```python
from build123d import *

# Parameters (mm, degrees)
SM_BASE_FLANGE_1_DEPTH = 910
SKETCH_6_W             = 17
SKETCH_6_H             = 97
CUT_EXTRUDE_1_DEPTH    = 24
SKETCH_7_W             = 101
SKETCH_7_H             = 35
CUT_EXTRUDE_2_DEPTH    = 59
CUT_EXTRUDE_3_DEPTH    = 10
SKETCH_9_R             = 3.5
SKETCH_9_R_2           = 6
CUT_EXTRUDE_3433_DEPTH = 10
SKETCH_10_R            = 3.25
SKETCH_10_R_2          = 6.5
CUT_EXTRUDE_5_DEPTH    = 10
SKETCH_11_R            = 2.5
CUT_EXTRUDE_6_DEPTH    = 10
SKETCH_12_R            = 3.25
CUT_EXTRUDE_7_DEPTH    = 10
SKETCH_13_R            = 2.5
CUT_EXTRUDE_8_DEPTH    = 10
SKETCH_16_R            = 2.5
CUT_EXTRUDE_11_DEPTH   = 10


# Sheet-metal steps are written as plain solids
with BuildPart() as part:
    # Sketch 1 → Базовая кромка1 (new, symmetric)
    with BuildSketch(Plane.XY):
        with BuildLine():
            Line((0, 0), (0, 18))
            ThreePointArc((0, 18), (-0.585786438, 19.414213562), (-2, 20))
            Line((-2, 20), (-11, 20))
            ThreePointArc((-11, 20), (-13.828427125, 21.171572875), (-15, 24))
            Line((-15, 24), (-15, 81))
            ThreePointArc((-15, 81), (-13.828427125, 83.828427125), (-11, 85))
            Line((-11, 85), (75.5, 85))
            ThreePointArc((75.5, 85), (78.328427125, 83.828427125), (79.5, 81))
            Line((79.5, 81), (79.5, 54))
            ThreePointArc((79.5, 54), (80.085786438, 52.585786438), (81.5, 52))
            Line((81.5, 52), (130.5, 52))
            ThreePointArc((130.5, 52), (131.914213562, 52.585786438), (132.5, 54))
            Line((132.5, 54), (132.5, 65))
            Line((132.5, 65), (134.5, 65))
            Line((134.5, 65), (134.5, 54))
            ThreePointArc((134.5, 54), (133.328427125, 51.171572875), (130.5, 50))
            Line((130.5, 50), (81.5, 50))
            ThreePointArc((81.5, 50), (78.671572875, 51.171572875), (77.5, 54))
            Line((77.5, 54), (77.5, 81))
            ThreePointArc((77.5, 81), (76.914213562, 82.414213562), (75.5, 83))
            Line((75.5, 83), (-11, 83))
            ThreePointArc((-11, 83), (-12.414213562, 82.414213562), (-13, 81))
            Line((-13, 81), (-13, 24))
            ThreePointArc((-13, 24), (-12.414213562, 22.585786438), (-11, 22))
            Line((-11, 22), (-2, 22))
            ThreePointArc((-2, 22), (0.828427125, 20.828427125), (2, 18))
            Line((2, 18), (2, 0))
            Line((2, 0), (0, 0))
        make_face()
    extrude(amount=SM_BASE_FLANGE_1_DEPTH, both=True)

    # Эскиз6 → Вырез-Вытянуть1 (cut)
    with BuildSketch(Plane.XZ):
        with Locations((-6.5, 861.5)):
            Rectangle(SKETCH_6_W, SKETCH_6_H)
        with Locations((-6.5, -861.5)):
            Rectangle(SKETCH_6_W, SKETCH_6_H)
    extrude(amount=-CUT_EXTRUDE_1_DEPTH, mode=Mode.SUBTRACT)

    # Эскиз7 → Вырез-Вытянуть2 (cut)
    with BuildSketch(Plane(origin=(134.5, 0, 0), x_dir=(0, 0, -1), z_dir=(1, 0, 0))):
        with Locations((859.5, 67.5)):
            Rectangle(SKETCH_7_W, SKETCH_7_H)
        with Locations((-859.5, 67.5)):
            Rectangle(SKETCH_7_W, SKETCH_7_H)
    extrude(amount=-CUT_EXTRUDE_2_DEPTH, mode=Mode.SUBTRACT)

    # Эскиз8 → Вырез-Вытянуть3 (cut)
    with BuildSketch(Plane.ZY.offset(15)):
        with BuildLine():
            Line((-5.5, 38), (-5.5, 67))
            ThreePointArc((-5.5, 67), (0, 72.5), (5.5, 67))
            Line((5.5, 67), (5.5, 38))
            ThreePointArc((5.5, 38), (0, 32.5), (-5.5, 38))
        make_face()
        with BuildLine():
            Line((-725.5, 38), (-725.5, 67))
            ThreePointArc((-725.5, 67), (-720, 72.5), (-714.5, 67))
            Line((-714.5, 67), (-714.5, 38))
            ThreePointArc((-714.5, 38), (-720, 32.5), (-725.5, 38))
        make_face()
        with BuildLine():
            Line((714.5, 38), (714.5, 67))
            ThreePointArc((714.5, 67), (720, 72.5), (725.5, 67))
            Line((725.5, 67), (725.5, 38))
            ThreePointArc((725.5, 38), (720, 32.5), (714.5, 38))
        make_face()
    extrude(amount=-CUT_EXTRUDE_3_DEPTH, mode=Mode.SUBTRACT)

    # Эскиз9 → Cut-Extrude 3433 (cut)
    with BuildSketch(Plane.XZ.offset(-50)):
        with Locations((106, 194)):
            Circle(SKETCH_9_R)
        with Locations((106, 144)):
            Circle(SKETCH_9_R)
        with Locations((106, 35)):
            Circle(SKETCH_9_R_2)
        with Locations((106, -761)):
            Circle(SKETCH_9_R_2)
        with BuildLine():
            Line((89, 90.5), (123, 90.5))
            ThreePointArc((123, 90.5), (128.5, 85), (123, 79.5))
            Line((123, 79.5), (89, 79.5))
            ThreePointArc((89, 79.5), (83.5, 85), (89, 90.5))
        make_face()
        with BuildLine():
            Line((89, 260.5), (123, 260.5))
            ThreePointArc((123, 260.5), (128.5, 255), (123, 249.5))
            Line((123, 249.5), (89, 249.5))
            ThreePointArc((89, 249.5), (83.5, 255), (89, 260.5))
        make_face()
        with BuildLine():
            Line((89, -360.5), (123, -360.5))
            ThreePointArc((123, -360.5), (128.5, -366), (123, -371.5))
            Line((123, -371.5), (89, -371.5))
            ThreePointArc((89, -371.5), (83.5, -366), (89, -360.5))
        make_face()
        with BuildLine():
            Line((89, -470.5), (123, -470.5))
            ThreePointArc((123, -470.5), (128.5, -476), (123, -481.5))
            Line((123, -481.5), (89, -481.5))
            ThreePointArc((89, -481.5), (83.5, -476), (89, -470.5))
        make_face()
        with BuildLine():
            Line((89, -620.5), (123, -620.5))
            ThreePointArc((123, -620.5), (128.5, -626), (123, -631.5))
            Line((123, -631.5), (89, -631.5))
            ThreePointArc((89, -631.5), (83.5, -626), (89, -620.5))
        make_face()
        with BuildLine():
            Line((89, -730.5), (123, -730.5))
            ThreePointArc((123, -730.5), (128.5, -736), (123, -741.5))
            Line((123, -741.5), (89, -741.5))
            ThreePointArc((89, -741.5), (83.5, -736), (89, -730.5))
        make_face()
    extrude(amount=-CUT_EXTRUDE_3433_DEPTH, mode=Mode.SUBTRACT)

    # Эскиз10 → Вырез-Вытянуть5 (cut)
    with BuildSketch(Plane(origin=(0, 85, 0), x_dir=(1, 0, 0), z_dir=(0, 1, 0))):
        with Locations(Location((20, 890, 0), (0, 0, 180))):
            Circle(SKETCH_10_R)
        with Locations(Location((20, 860, 0), (0, 0, 180))):
            Circle(SKETCH_10_R_2)
        with Locations(Location((20, 840, 0), (0, 0, 180))):
            Circle(SKETCH_10_R)
        with Locations(Location((60, 860, 0), (0, 0, 180))):
            Circle(SKETCH_10_R_2)
        with Locations(Location((20, 770, 0), (0, 0, 180))):
            Circle(SKETCH_10_R)
        with Locations((20, -770)):
            Circle(SKETCH_10_R)
        with Locations((60, -860)):
            Circle(SKETCH_10_R_2)
        with Locations((20, -840)):
            Circle(SKETCH_10_R)
        with Locations((20, -860)):
            Circle(SKETCH_10_R_2)
        with Locations((20, -890)):
            Circle(SKETCH_10_R)
    cut_extrude_5 = extrude(amount=-CUT_EXTRUDE_5_DEPTH, mode=Mode.SUBTRACT)

    # Зеркальное отражение1: Вырез-Вытянуть5 across plane
    add(cut_extrude_5.mirror(Plane(origin=(35, 35, 0), x_dir=(0, 0, 1), z_dir=(-0.7071067811865499, -0.7071067811865452, 0))), mode=Mode.SUBTRACT)

    # Эскиз11 → Вырез-Вытянуть6 (cut)
    with BuildSketch(Plane.ZY):
        with Locations((-797, 7)):
            Circle(SKETCH_11_R)
        with Locations((797, 7)):
            Circle(SKETCH_11_R)
    extrude(amount=-CUT_EXTRUDE_6_DEPTH, mode=Mode.SUBTRACT)

    # Эскиз12 → Вырез-Вытянуть7 (cut)
    with BuildSketch(Plane.XZ.offset(-50)):
        with Locations((92.5, 797)):
            Circle(SKETCH_12_R)
        with Locations((119.5, 797)):
            Circle(SKETCH_12_R)
        with Locations(Location((119.5, -797, 0), (0, 0, 180))):
            Circle(SKETCH_12_R)
        with Locations(Location((92.5, -797, 0), (0, 0, 180))):
            Circle(SKETCH_12_R)
    extrude(amount=-CUT_EXTRUDE_7_DEPTH, mode=Mode.SUBTRACT)

    # Эскиз13 → Вырез-Вытянуть8 (cut)
    with BuildSketch(Plane(origin=(2, 0, 0), x_dir=(0, 0, -1), z_dir=(1, 0, 0))):
        with Locations((775, 10)):
            Circle(SKETCH_13_R)
        with Locations((750, 10)):
            Circle(SKETCH_13_R)
        with Locations((725, 10)):
            Circle(SKETCH_13_R)
        with Locations((700, 10)):
            Circle(SKETCH_13_R)
        with Locations((650, 10)):
            Circle(SKETCH_13_R)
        with Locations((600, 10)):
            Circle(SKETCH_13_R)
        with Locations((550, 10)):
            Circle(SKETCH_13_R)
        with Locations((500, 10)):
            Circle(SKETCH_13_R)
        with Locations((450, 10)):
            Circle(SKETCH_13_R)
        with Locations((400, 10)):
            Circle(SKETCH_13_R)
        with Locations((350, 10)):
            Circle(SKETCH_13_R)
        with Locations((300, 10)):
            Circle(SKETCH_13_R)
        with Locations((250, 10)):
            Circle(SKETCH_13_R)
        with Locations((200, 10)):
            Circle(SKETCH_13_R)
        with Locations((150, 10)):
            Circle(SKETCH_13_R)
        with Locations((100, 10)):
            Circle(SKETCH_13_R)
        with Locations((50, 10)):
            Circle(SKETCH_13_R)
        with Locations((0, 10)):
            Circle(SKETCH_13_R)
        with Locations((-50, 10)):
            Circle(SKETCH_13_R)
        with Locations((-100, 10)):
            Circle(SKETCH_13_R)
        with Locations((-150, 10)):
            Circle(SKETCH_13_R)
        with Locations((-200, 10)):
            Circle(SKETCH_13_R)
        with Locations((-775, 10)):
            Circle(SKETCH_13_R)
        with Locations((-750, 10)):
            Circle(SKETCH_13_R)
        with Locations((-725, 10)):
            Circle(SKETCH_13_R)
        with Locations((-700, 10)):
            Circle(SKETCH_13_R)
        with Locations((-250, 10)):
            Circle(SKETCH_13_R)
        with Locations((-300, 10)):
            Circle(SKETCH_13_R)
        with Locations((-350, 10)):
            Circle(SKETCH_13_R)
        with Locations((-400, 10)):
            Circle(SKETCH_13_R)
        with Locations((-450, 10)):
            Circle(SKETCH_13_R)
    extrude(amount=-CUT_EXTRUDE_8_DEPTH, mode=Mode.SUBTRACT)

    # Эскиз16 → Вырез-Вытянуть11 (cut)
    with BuildSketch(Plane(origin=(0, 52, 0), x_dir=(1, 0, 0), z_dir=(0, 1, 0))):
        with Locations(Location((109.5, 579, 0), (0, 0, 180))):
            Circle(SKETCH_16_R)
        with Locations(Location((109.5, 554, 0), (0, 0, 180))):
            Circle(SKETCH_16_R)
        with Locations(Location((109.5, 223.5, 0), (0, 0, 180))):
            Circle(SKETCH_16_R)
        with Locations(Location((109.5, 198.5, 0), (0, 0, 180))):
            Circle(SKETCH_16_R)
        with Locations(Location((109.5, -156.5, 0), (0, 0, 180))):
            Circle(SKETCH_16_R)
        with Locations(Location((109.5, -181.5, 0), (0, 0, 180))):
            Circle(SKETCH_16_R)
    extrude(amount=-CUT_EXTRUDE_11_DEPTH, mode=Mode.SUBTRACT)


solid = part.part
```
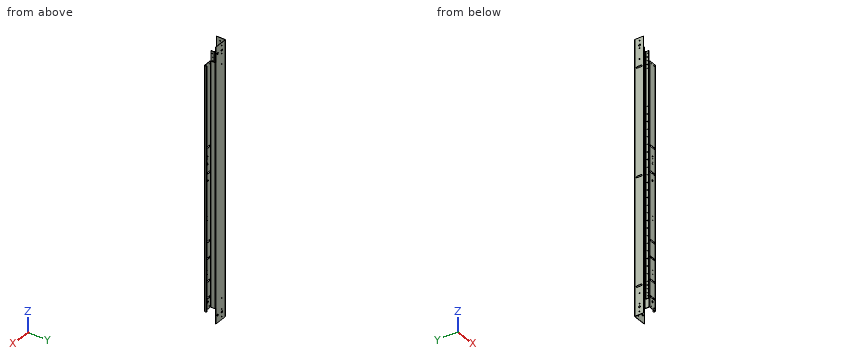
The model under review builds one solid part; all positions refer to its coordinate system, in mm. Round coordinates to 2 decimals unless told otherwise and drop trailing zeros. Order: outer loops, then holes, each group sorted by start corner. A loop starts at its lowest first (then second) coordinate and runs counter-clockwise, first axis right, second up.
(1) For P1, Ø2, axis at x = 95, z = -698, coming from the -Y side; P2, Ø6, axis at x = 5, y = 24.5, coming from the +Z side; P3, Ø6, axis at y = 10, z = -775, coming from the +X side; P4, Ø12, axis at y = 34, z = 507, coming from the +X side, all flat-tipped, find the tip position at first contact; note any pin that passes through.
Working result:
P1: stops at y = 50
P2: passes through
P3: stops at x = 2
P4: stops at x = -13
(2) Wall thickness on L1, parallel to X at y = 55, z = -391; L2, parallel to X at y = 50.5, z = 797; L3, parallel to X at y = 73, z = 596.5: over which ranges is each line inside the solid? List them lowest first.
Working result:
L1: x = -15 to -13, 77.5 to 79.5, 132.5 to 134.5
L2: x = -15 to -13, 79.56 to 89.25, 95.75 to 116.25, 122.75 to 132.44
L3: x = -15 to -13, 77.5 to 79.5
(3) Take a section at A-A, the plane z = 601.5. State the section outline as (x, y) points, plus the area to 3 significant figures.
Working result:
outline: (-15, 24) arc R4 ccw to (-11, 20) - (-2, 20) arc R2 cw to (0, 18) - (0, 0) - (2, 0) - (2, 18) arc R4 ccw to (-2, 22) - (-11, 22) arc R2 cw to (-13, 24) - (-13, 81) arc R2 cw to (-11, 83) - (75.5, 83) arc R2 cw to (77.5, 81) - (77.5, 54) arc R4 ccw to (81.5, 50) - (130.5, 50) arc R4 ccw to (134.5, 54) - (134.5, 65) - (132.5, 65) - (132.5, 54) arc R2 cw to (130.5, 52) - (81.5, 52) arc R2 cw to (79.5, 54) - (79.5, 81) arc R4 ccw to (75.5, 85) - (-11, 85) arc R4 ccw to (-15, 81) - close
area: 572 mm2
